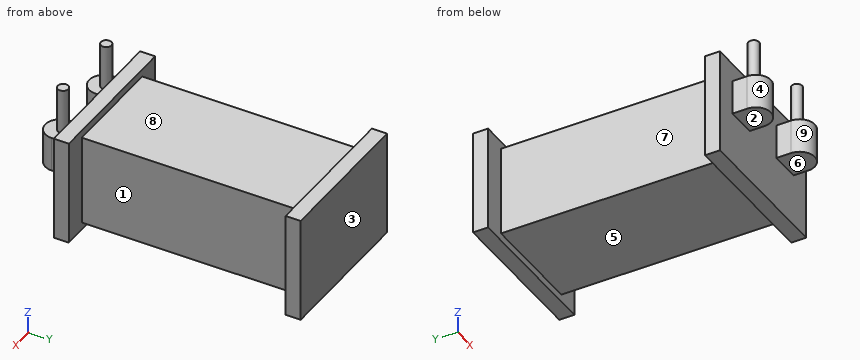
```python
from build123d import *

# Parameters (mm, degrees)
SKETCH250_W  = 7
SKETCH250_H  = 14.4
PAD172_DEPTH = 3
SKETCH256_W  = 10
SKETCH256_H  = 7
PAD182_DEPTH = 1
SKETCH253_W  = 10
SKETCH253_H  = 7
PAD175_DEPTH = 1
PAD171_DEPTH = 2.3
SKETCH251_R  = 0.35
PAD183_DEPTH = 3


with BuildPart() as part:
    # Sketch250 → Pad172 (new body, symmetric)
    with BuildSketch(Plane.XY):
        with Locations((0, -0.37169)):
            Rectangle(SKETCH250_W, SKETCH250_H)
    extrude(amount=PAD172_DEPTH, both=True)

    # Sketch256 (on Face3 of Pad172) → Pad182 (join)
    with BuildSketch(Plane.XZ.offset(7.57169)):
        Rectangle(SKETCH256_W, SKETCH256_H)
    extrude(amount=PAD182_DEPTH)

    # Sketch253 (on Face11 of Pad182) → Pad175 (join)
    with BuildSketch(Plane(origin=(0, 6.82831, 0), x_dir=(-1, 0, 0), z_dir=(0, 1, 0))):
        Rectangle(SKETCH253_W, SKETCH253_H)
    extrude(amount=PAD175_DEPTH)

    # Sketch260 → Pad171 (join)
    with BuildSketch(Plane.XY):
        with BuildLine():
            ThreePointArc((-3.539731, -9.545275), (-2.539731, -10.545275), (-1.539731, -9.545275))
            Line((-1.539731, -8.57169), (-1.539731, -9.545275))
            Line((-3.539731, -8.57169), (-1.539731, -8.57169))
            Line((-3.539731, -8.57169), (-3.539731, -9.545275))
        make_face()
        with BuildLine():
            ThreePointArc((1.539731, -9.545275), (2.539731, -10.545275), (3.539731, -9.545275))
            Line((3.539731, -8.57169), (3.539731, -9.545275))
            Line((3.539731, -8.57169), (1.539731, -8.57169))
            Line((1.539731, -8.57169), (1.539731, -9.545275))
        make_face()
    extrude(amount=PAD171_DEPTH)

    # Sketch251 (on Face19 of Pad171) → Pad183 (join)
    with BuildSketch(Plane.XY.offset(2.3)):
        with Locations((-2.5, -9.384607)):
            Circle(SKETCH251_R)
        with Locations((2.5, -9.384607)):
            Circle(SKETCH251_R)
    extrude(amount=PAD183_DEPTH)


with BuildPart() as part_1:
    # Body052 placement: moved
    add(part.part.moved(Location((3.5, -13, 0))))


solid = part_1.part
```
CAD build for the part. Positions are in the model's coordinates, mm. Face numbers are marked on the shaded views. A direction names the side the tool comes from. Round coordinates to 2 decimals unless told otherwise and drop trailing zeros. Loops run counter-clockwise (first coordinate to the right, second up) from the corner with the lowest first, then second, coordinate; pieces in that order, holes last. Notation, with made-up numbers: M 74.25,61.25 L 117.25,61.25 A29 ccw 117.25,84.25 Z; hole C 87.5,21 d4. An arc over 180 degrees is marked long. Use a Markdown table: item, result. Add a question column.
(1) Cut at A-A (z = 1). Give the cut face in (x, y).
(2) Drill centre lines: line 1 (Y direction, x = -0.25, z = 3); line 2 (Y direction, x = 3.5, z = 2); line 3 (Z direction, x = 1, y = -12). Where is each one in solid material? Low to high.
(3) Cut at B-B (x = 3.5). Give the cut face in (y, z).
(4) Pull direction Y, two halves, no side cores. Call the marked faces 1, 2, 3 and 4: +Y half, -Y half, draft (parallel to the pull), parting line (faces both ways), or undercut.
(5) Which spindle directions (+Z, -Z, +X, -X, +Y, -Y) get a long thin tool onto all of the face, cutting with end or side? Do the marked faces 5, 6, 7, 8 and 9. Say none if no direction does.
(6) Flat gauge pins, fed straight in: pin 1 (3.5 mm diameter, centred on x = 3.5, y = -10.5, fed in from +Z); pin 2 (1 mm diameter, centred on x = 4, y = -12.5, fed in from -Z); pin 3 (5 mm diameter, centred on y = -12, z = 1.5, fed in from +X). Where does each tip first touch, or does it go through?
(7) Cut at C-C (y = -16). Give the cut face in (x, z), and give its area (3 significant figures).
(8) Cut at D-D (z = 3.75). Give the cut face in (x, y), and give its area (3 significant figures).
Geometry says:
| question | item | result |
|---|---|---|
| 1 | outline | M -1.5,-21.57 L -0.04,-21.57 L -0.04,-22.55 A1 ccw 1.96,-22.55 L 1.96,-21.57 L 5.04,-21.57 L 5.04,-22.55 A1 ccw 7.04,-22.55 L 7.04,-21.57 L 8.5,-21.57 L 8.5,-20.57 L 7,-20.57 L 7,-6.17 L 8.5,-6.17 L 8.5,-5.17 L -1.5,-5.17 L -1.5,-6.17 L 0,-6.17 L 0,-20.57 L -1.5,-20.57 Z |
| 2 | line 1 | y = -21.57 to -20.57, -6.17 to -5.17 |
| 2 | line 2 | y = -21.57 to -5.17 |
| 2 | line 3 | z = -3 to 3 |
| 3 | outline | M -21.57,-3.5 L -20.57,-3.5 L -20.57,-3 L -6.17,-3 L -6.17,-3.5 L -5.17,-3.5 L -5.17,3.5 L -6.17,3.5 L -6.17,3 L -20.57,3 L -20.57,3.5 L -21.57,3.5 Z |
| 4 | face 1 | undercut |
| 4 | face 2 | draft |
| 4 | face 3 | +Y half |
| 4 | face 4 | -Y half |
| 5 | face 5 | -Z, +X, -X |
| 5 | face 6 | -Z, +X, -X, -Y |
| 5 | face 7 | +Z, -Z, -X |
| 5 | face 8 | +Z, +X, -X |
| 5 | face 9 | +Z, -Z, -Y |
| 6 | pin 1 | stops at z = 3 |
| 6 | pin 2 | stops at z = -3 |
| 6 | pin 3 | stops at x = 7 |
| 7 | outline | M 0,-3 L 7,-3 L 7,3 L 0,3 Z |
| 7 | area | 42.0 mm² |
| 8 | outline | C 1,-22.38 d0.7; C 6,-22.38 d0.7 |
| 8 | area | 0.770 mm² |
